Design review of the part built by this model. Coordinates are the model's own, in mm. A direction names the side the tool comes from. Coordinates: 2 decimals unless noted, no trailing zeros. Loops run counter-clockwise (first coordinate to the right, second up) from the corner with the lowest first, then second, coordinate; pieces in that order, holes last. Notation, with made-up numbers: (-32.75, -36.75) -> (-19.75, -36.75) arc R8 cw to (-19.75, -32.75) -> close; hole circle Ø7 at (-6.5, -7.5). An arc over 180 degrees is marked (long way). Answer as a JSON object with one key per item and string values.
```python
from build123d import *
from OCP.BRepFilletAPI import BRepFilletAPI_MakeChamfer

# Parameters (mm, degrees)
BOSS_EXTRUDE1_DEPTH = 5
CHAMFER1_SIZE       = 4
CHAMFER1_SIZE2      = 14.92820323
CHAMFER2_SIZE       = 3
CHAMFER2_SIZE2      = 7.42526056


with BuildPart() as part:
    # Sketch1 → Boss-Extrude1 (new body)
    with BuildSketch(Plane(origin=(0, 0, 0), x_dir=(1, 0, 0), z_dir=(0, 1, 0))):
        Polygon((-7.5, 40), (7.5, 40), (7.5, -40), (1, -40), (1, -35), (-1, -35), (-1, -40), (-7.5, -40), align=None)
        with BuildLine():
            Line((-2.5, -30), (-2.5, 5))
            ThreePointArc((-2.5, 5), (0, 7.5), (2.5, 5))
            Line((2.5, 5), (2.5, -30))
            ThreePointArc((2.5, -30), (0, -32.5), (-2.5, -30))
        make_face(mode=Mode.SUBTRACT)
    extrude(amount=BOSS_EXTRUDE1_DEPTH)

    # Chamfer1: one chamfer whose edges measure the first distance from different faces: ONE call of the kernel's chamfer builder (chamfer() names one face for all edges)
    chamfer1_edges_1 = [part.edges().sort_by_distance(p)[0] for p in [
        (-7.5, 2.5, 40),
    ]]
    chamfer1_side_1 = [part.faces().sort_by_distance(p)[0] for p in [
        (-4.25, 2.5, 40),
    ]]
    chamfer1_edges_2 = [part.edges().sort_by_distance(p)[0] for p in [
        (7.5, 2.5, 40),
    ]]
    chamfer1_side_2 = [part.faces().sort_by_distance(p)[0] for p in [
        (4.25, 2.5, 40),
    ]]
    chamfer1 = BRepFilletAPI_MakeChamfer(part.part.solid().wrapped)
    for e in chamfer1_edges_1:
        chamfer1.Add(CHAMFER1_SIZE, CHAMFER1_SIZE2, e.wrapped, chamfer1_side_1[0].wrapped)  # the first distance lies on this face
    for e in chamfer1_edges_2:
        chamfer1.Add(CHAMFER1_SIZE, CHAMFER1_SIZE2, e.wrapped, chamfer1_side_2[0].wrapped)  # the first distance lies on this face
    add(Compound.cast(chamfer1.Shape()), mode=Mode.REPLACE)

    # Chamfer2
    chamfer2_edges = [part.edges().sort_by_distance(p)[0] for p in [
        (2.25, 5, 40),
    ]]
    chamfer2_side = [part.faces().sort_by_distance(p)[0] for p in [
        (2.25, 2.5, 40),
    ]]
    chamfer(chamfer2_edges, length=CHAMFER2_SIZE, length2=CHAMFER2_SIZE2, reference=chamfer2_side[0])


solid = part.part
```
1) Add section A-A, the plane z = 8.5. Give the boundary of the cut face in (x, y), and give its area (3 significant figures).
Completed:
{"outline": "(-7.5, 0) -> (-2.5, 0) -> (-2.5, 5) -> (-7.5, 5) -> close; (2.5, 0) -> (7.5, 0) -> (7.5, 5) -> (2.5, 5) -> close", "area": "50.0 mm²"}
2) Clearance check with a flat-ended pin moving along its axis: pin 1 Ø1.2 at (y, z) = (1, 38.5) entering from -X. State where the tip first meets the part, or that it passes through.
Completed:
{"pin 1": "x = -4.06"}
3) The part is to be moulded in two halves that separate along Z. For faces 4 (the flat face through (-2, 1, 40)), 5 (the cylindrical face through (-0.1, 2.5, -7.5)), 6 (the flat face through (-7.5, 2, -7)), say which applies: pulls with the +Z half, pulls with the -Z half, needs draft (parallel to the pull), parting line crosses it, or undercut.
Completed:
{"face 4": "pulls with the +Z half", "face 5": "undercut", "face 6": "needs draft"}
4) Add section B-B, the plane x = 0. Give the boundary of the cut face in (y, z).
Completed:
{"outline": "(0, -40) -> (5, -40) -> (5, -7.5) -> (0, -7.5) -> close; (0, 32.5) -> (5, 32.5) -> (5, 32.57) -> (4.02, 35) -> (0, 35) -> close"}
5) For faces 1 (the flat face through (0, 2, 35)), 2 (the flat face through (0.077, 4.188, 34.585)), 3 (the flat face through (-2.5, 2, 13)), list the 3-axis set-ups (+Z, -Z, +X, -X, +Y, -Y) from which the entire face can be reached by the end or side of a thin tool; tool diameter is ignored.
Completed:
{"face 1": "+Z, +Y, -Y", "face 2": "+Z, +X, -X, +Y", "face 3": "+Y, -Y"}
6) Add section C-C, the plane y = 2.95. Give the boundary of the cut face in (x, z).
Completed:
{"outline": "(-7.5, -40) -> (7.5, -40) -> (7.5, 25.07) -> (4.13, 37.65) -> (1, 37.65) -> (1, 35) -> (-1, 35) -> (-1, 37.65) -> (-4.13, 37.65) -> (-7.5, 25.07) -> close; hole (-2.5, -5) arc R2.5 ccw to (2.5, -5) -> (2.5, 30) arc R2.5 ccw to (-2.5, 30) -> close"}
7) Wall thickness on probe 1 along Z at (x, y) = (0, 1.3); probe 2 along X at (y, z) = (0.9, 12); probe 3 along X at (y, z) = (3.55, 36): over which ranges is each line inside the solid? List them lowest first.
Completed:
{"probe 1": "-40 to -7.5, 32.5 to 35", "probe 2": "-7.5 to -2.5, 2.5 to 7.5", "probe 3": "-4.57 to -1, 1 to 4.57"}
8) Add section D-D, the plane z = 27. Give the boundary of the cut face in (x, y), and give its area (3 significant figures).
Completed:
{"outline": "(-6.98, 0) -> (-2.5, 0) -> (-2.5, 5) -> (-6.98, 5) -> close; (2.5, 0) -> (6.98, 0) -> (6.98, 5) -> (2.5, 5) -> close", "area": "44.8 mm²"}
